The listing builds one solid part. Answer for the finished solid, in the listing's coordinates (mm). A direction names the side the tool comes from. Coordinates: 2 decimals unless noted, no trailing zeros. Order: outer loops, then holes, each group sorted by start corner. A loop starts at its lowest first (then second) coordinate and runs counter-clockwise, first axis right, second up. Notation, with made-up numbers: (7, -26) -> (13, -26) arc R23 cw to (13, 8) -> close; hole circle Ø9 at (81.25, -22). An arc over 180 degrees is marked (long way). Return JSON: item names as keys, results as strings.
from build123d import *

# Parameters (mm, degrees)
ESQUISSE1_W                                 = 100
ESQUISSE1_H                                 = 20
BOSS_EXTRU_1_DEPTH                          = 25
FRAISAGE_POUR_VIS_T_TE_FRAIS_E_M81_AT_COUNT = 2
FRAISAGE_POUR_VIS_T_TE_FRAIS_E_M81_AT_PITCH = 48
DIAM_TRE_DU_PER_AGE_8_0_8_1_D               = 8
ENL_V_MAT_EXTRU_1_DEPTH                     = 51


with BuildPart() as part:
    # Esquisse1 → Boss.-Extru.1 (new body, symmetric)
    with BuildSketch(Plane.XY):
        Rectangle(ESQUISSE1_W, ESQUISSE1_H)
    extrude(amount=BOSS_EXTRU_1_DEPTH, both=True)

    # Esquisse13 → Fraisage pour vis à tête fraisée M81 (revolve, cut)
    with BuildSketch(Plane(origin=(-24, -10, 0), x_dir=(0, 0, -1), z_dir=(1, 0, 0))):
        Polygon((0, 0), (0, 20), (4, 20), (4, 14), (8, 10), (8, 0), align=None)
    fraisage_pour_vis_t_te_frais_e_m81 = revolve(axis=Axis((-24, -16.35, 0), (0, 1, 0)), mode=Mode.SUBTRACT)

    # Fraisage pour vis à tête fraisée M81 at: Fraisage pour vis à tête fraisée M81 ×2
    with Locations(*[(i * FRAISAGE_POUR_VIS_T_TE_FRAIS_E_M81_AT_PITCH, 0, 0) for i in range(1, FRAISAGE_POUR_VIS_T_TE_FRAIS_E_M81_AT_COUNT)]):
        add(fraisage_pour_vis_t_te_frais_e_m81, mode=Mode.SUBTRACT)

    # Diamètre du perçage Ø8.0 (8)1 (through all)
    with Locations(Plane(origin=(0, -10, 0), x_dir=(-1, 0, 0), z_dir=(0, -1, 0))):
        with Locations((-40, 0), (40, 0)):
            Hole(DIAM_TRE_DU_PER_AGE_8_0_8_1_D / 2)

    # Esquisse16 → Enlèv. mat.-Extru.1 (cut, through all)
    with BuildSketch(Plane(origin=(0, 0, -25), x_dir=(-1, 0, 0), z_dir=(0, 0, -1))):
        Polygon((0, 2), (-50, -5.027041735), (-50, -10), (50, -10), (50, -5.027041735), align=None)
    extrude(amount=-ENL_V_MAT_EXTRU_1_DEPTH, mode=Mode.SUBTRACT)


solid = part.part
1. The part is cut by section A-A on y = 6.25. Give the vertices of the cut face in (x, z), and give its area (3 significant figures).
Answer block:
{"outline": "(-50, -25) -> (50, -25) -> (50, 25) -> (-50, 25) -> close; hole circle Ø8 at (-40, 0); hole circle Ø8 at (-24, 0); hole circle Ø8 at (24, 0); hole circle Ø8 at (40, 0)", "area": "4,800 mm2"}
2. Consider line 1 (Z direction, x = -24, y = 5.8); line 2 (Y direction, x = 44, z = -21); line 3 (Z direction, x = -43.5, y = 1.5). Determine where each line is inside the solid, lowest interval first. Write a range as from..to.
Answer block:
{"line 1": "z = -25..-4, 4..25", "line 2": "y = -4.18..10", "line 3": "z = -25..-1.94, 1.94..25"}
3. The part is cut by section C-C on z = 0. Give the number of separate pieces and of enclosed holes in the cut face, and give its area (3 significant figures).
Answer block:
{"separate pieces": "5", "enclosed holes": "0", "area": "697 mm2"}
4. The part is cut by section B-B on x = 40. Give the vertices of the cut face in (y, z), and give its area (3 significant figures).
Answer block:
{"outline": "(-3.62, -25) -> (10, -25) -> (10, -4) -> (-3.62, -4) -> close; (-3.62, 4) -> (10, 4) -> (10, 25) -> (-3.62, 25) -> close", "area": "572 mm2"}
5. The part is cut by section D-D on x = 24. Give the vertices of the cut face in (y, z).
Answer block:
{"outline": "(-1.37, -25) -> (10, -25) -> (10, -4) -> (4, -4) -> (0, -8) -> (-1.37, -8) -> close; (-1.37, 8) -> (0, 8) -> (4, 4) -> (10, 4) -> (10, 25) -> (-1.37, 25) -> close"}
6. For faces 1 (the face through (-30.906, -2.343, -5.906)), 2 (the face through (-31.932, -0.989, 1.041)), 3 (the face through (-27.966, 6.958, 0.521)), determine the directions among +Z, -Z, +X, -X, +Y, -Y from which every point of the face is accessible in a straight line to the end or side of a thin tool.
Answer block:
{"face 1": "+Z, -Z, -Y", "face 2": "-Y", "face 3": "+Y, -Y"}
7. Each of these flat-tipped pins is pushed along its axis until it touches: pin 1 Ø13 at (x, z) = (-40, 0) entering from -Y; pin 2 Ø13 at (x, z) = (-24, 0) entering from -Y; pin 3 Ø5 at (x, z) = (-22, 1) entering from -Y. Where does it stop, or does it pass through?
Answer block:
{"pin 1": "stops at y = -4.54", "pin 2": "stops at y = 1.5", "pin 3": "stops at y = 3.26"}
